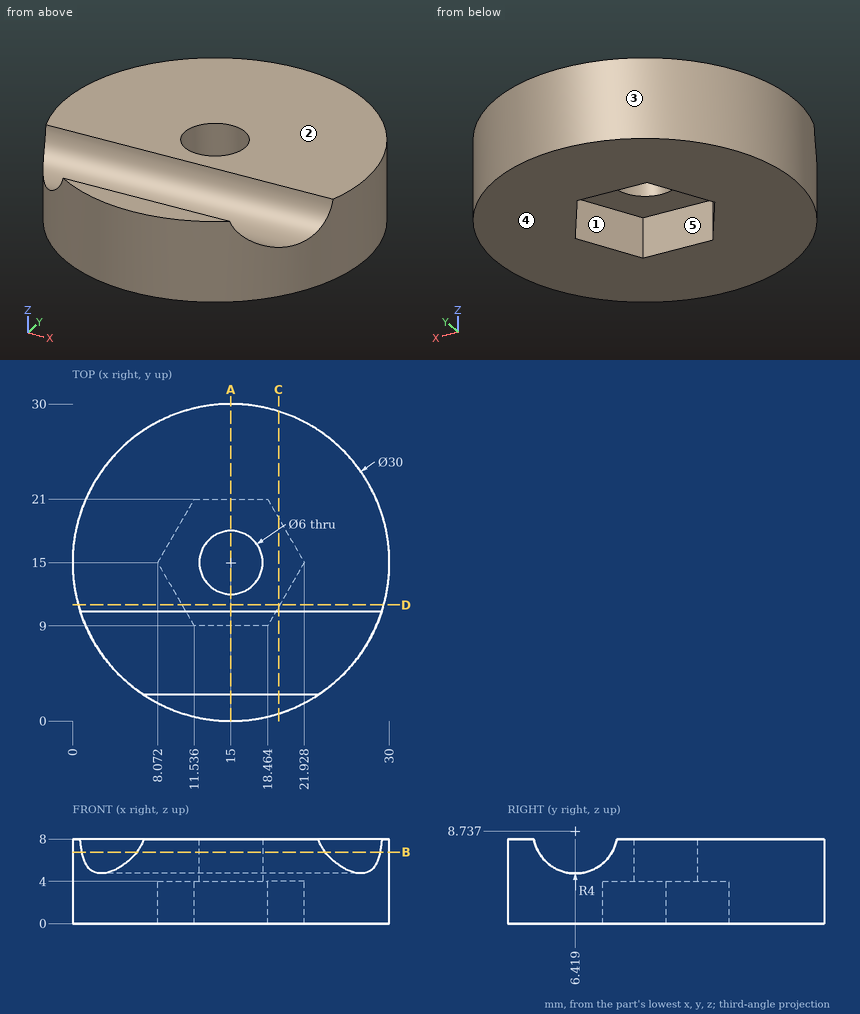
Input: dimensioned drawing with shaded views. Units: mm. Origin: part minimum x, y, z. A direction names the side the tool comes from. Coordinates: 2 decimals unless noted, no trailing zeros. Loops run counter-clockwise (first coordinate to the right, second up) from the corner with the lowest first, then second, coordinate; pieces in that order, holes last. Notation, with made-up numbers: M 10,-27.5 L 19,-27.5 A33 ccw 19,10.5 Z; hole C 68.25,75.5 d3. An arc over 180 degrees is marked long. Put each result on its own line as item: value.
(1) Draft query along Y for the marked faces 3, 4 and 5. Return one class per face: pulls with the +Y half, pulls with the -Y half, needs draft (parallel to the pull), parting line crosses it, or undercut.
Answer sheet:
face 3: parting line crosses it
face 4: needs draft
face 5: undercut
(2) Cut plane B-B on z = 6.75. Return the cut outline in (x, y), then the cut area to 3 significant figures.
Answer sheet:
outline: M 0.9,9.89 L 29.1,9.89 A15 ccw long Z; M 6.07,2.95 A15 ccw 23.93,2.95 Z; hole C 15,15 d6
area: 511 mm^2
(3) Material intervals for probe 1 along Y at (x, z) = (15, 7) (1 decimal); probe 2 along Y at (x, z) = (16, 7.75) (1 decimal); probe 3 along Y at (x, z) = (15, 2), sorted ascending.
Answer sheet:
probe 1: y = 0 to 2.8, 10 to 12, 18 to 30
probe 2: y = 0 to 2.5, 10.3 to 12.2, 17.8 to 30
probe 3: y = 0 to 9, 21 to 30
(4) Cut plane A-A on x = 15. Return the cut outline in (y, z).
Answer sheet:
outline: M 0,0 L 9,0 L 9,4 L 12,4 L 12,8 L 10.35,8 A4 cw 2.49,8 L 0,8 Z; M 18,4 L 21,4 L 21,0 L 30,0 L 30,8 L 18,8 Z
(5) Access query for the marked faces 1 and 2. Directions: +Z, -Z, +X, -X, +Y, -Y. A direction counts if a zero-diameter tool reaches every point of the face in a straight line with its end or side. Return the directions, or none.
Answer sheet:
face 1: -Z
face 2: +Z, +X, -X, +Y, -Y
(6) Cut plane D-D on y = 11. Return the cut outline in (x, z).
Answer sheet:
outline: M 0.54,0 L 10.38,0 L 10.38,4 L 19.62,4 L 19.62,0 L 29.46,0 L 29.46,8 L 0.54,8 Z
(7) Cut plane C-C on x = 19.5. Return the cut outline in (y, z).
Answer sheet:
outline: M 0.69,0 L 10.79,0 L 10.79,4 L 19.21,4 L 19.21,0 L 29.31,0 L 29.31,8 L 10.35,8 A4 cw 2.49,8 L 0.69,8 Z
(8) First-contact query: pin 1 (1.5 mm diameter, centred on x = 12.5, y = 3.5, fed in from +Z) (1 decimal); pin 2 (2 mm diameter, centred on y = 9.5, z = 5.5, fed in from +X); pin 3 (1 mm diameter, centred on x = 19.5, z = 7, fed in from -Y). Flat tips, straight axial feed; report the tip coordinate or a pass-through.
Answer sheet:
pin 1: stops at z = 7.1
pin 2: stops at x = 29.31
pin 3: stops at y = 0.54
